Answer from the drawing. Dimensions are ordinates in mm from the lowest x, y and z of the part. A direction names the side the tool comes from. Give positions to 0.01 mm unless a question says otherwise; leave off trailing zeros. Order: outer loops, then holes, each group sorted by start corner. A loop starts at its lowest first (then second) coordinate and runs counter-clockwise, first axis right, second up. Notation, with made-up numbers: (67, 36.25) -> (76, 36.25) arc R31 ccw to (76, 69.25) -> close; hole circle Ø6 at (-20.75, 73). An arc over 180 degrees is marked (long way). Write item = value, one per line. Start each with the question number.
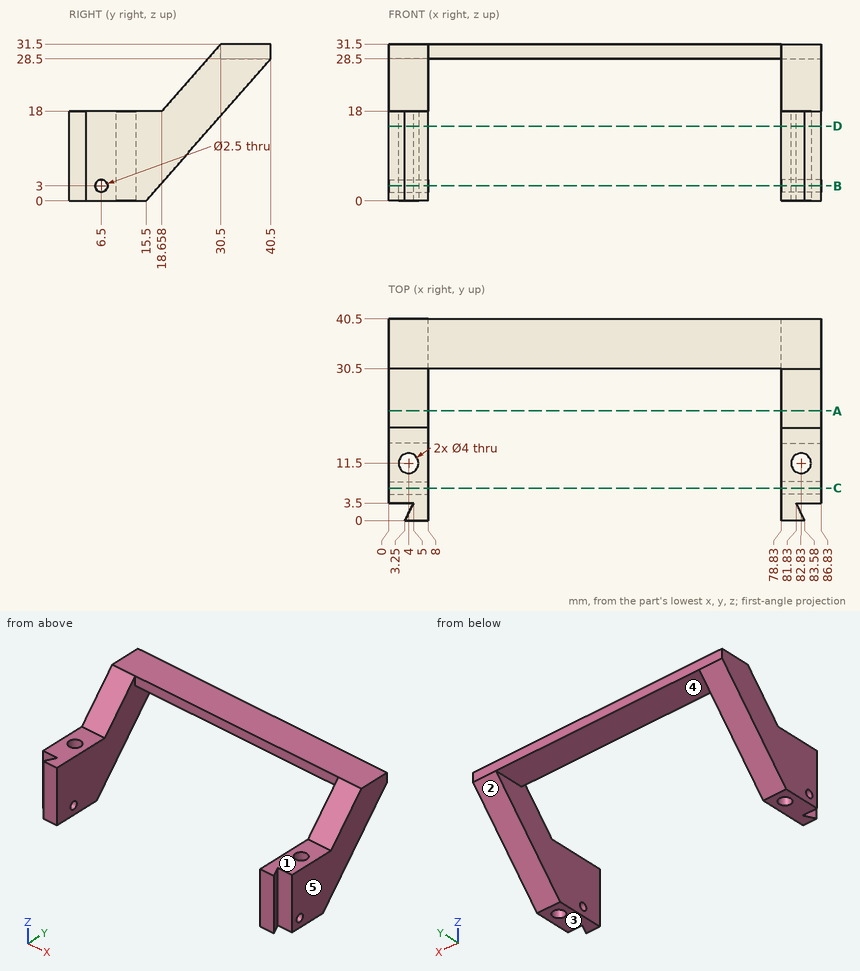
Item 1: Consider L1, parallel to Y at x = 82, z = 12; L2, parallel to X at y = 4, z = 2; L3, parallel to X at y = 12, z = 2. Determine where each line is inside the solid, lowest interval first. Write a range as from..to.
Item 2: A cutting plane is placed at A-A, the plane y = 22. Write down the section's boundary in (x, z), plus the area to 3 significant figures.
Item 3: A cutting plane is placed at C-C, the plane y = 6.5. Write down the section's boundary in (x, z).
Item 4: Flat-ended cylindrical pins translate along their axes: pin 1 (11 mm diameter, centred on x = 37.5, y = 34, fed in from -Z); pin 2 (6.5 mm diameter, centred on x = 84, y = 5.5, fed in from +Z); pin 3 (3.5 mm diameter, centred on x = 43.5, z = 29.5, fed in from -Y). Find the tip coordinate at first contact, or state that the pin passes through.
Item 5: Which of the six approach directions +Z, -Z, +X, -X, +Y, -Y give full straight-line access (tool end or side, diameter ignored) to the marked faces 1 and 2?
Item 6: A cutting plane is placed at B-B, the plane z = 3. Write down the section's boundary in (x, y), plus the area to 3 significant figures.
Item 7: The mould has two halves that part along X. Classify the marked faces 3, 4 and 5: +X half, -X half, draft (parallel to the pull), parting line (faces both ways), or undercut.
Item 8: A cutting plane is placed at D-D, the plane z = 15. Write down the section's boundary in (x, y).
Check values:
q1.L1 = 0..3.16, 3.5..9.68, 13.32..26.03
q1.L2 = 0..8, 78.83..86.83
q1.L3 = 0..2.06, 5.94..8, 78.83..80.89, 84.77..86.83
q2.outline = (0, 7.41) -> (8, 7.41) -> (8, 21.81) -> (0, 21.81) -> close; (78.83, 7.41) -> (86.83, 7.41) -> (86.83, 21.81) -> (78.83, 21.81) -> close
q2.area = 230 mm^2
q3.outline = (0, 0) -> (8, 0) -> (8, 1.75) -> (0, 1.75) -> close; (0, 4.25) -> (8, 4.25) -> (8, 18) -> (0, 18) -> close; (78.83, 0) -> (86.83, 0) -> (86.83, 1.75) -> (78.83, 1.75) -> close; (78.83, 4.25) -> (86.83, 4.25) -> (86.83, 18) -> (78.83, 18) -> close
q4.pin_1 = 28.5
q4.pin_2 = 18
q4.pin_3 = 30.5
q5.face_1 = +Z, +X, -X, -Y
q5.face_2 = -Z, +X, -X, +Y
q6.outline = (0, 3.5) -> (5, 3.5) -> (3.25, 0) -> (8, 0) -> (8, 5.25) -> (0, 5.25) -> close; (0, 7.75) -> (8, 7.75) -> (8, 18.13) -> (0, 18.13) -> close; (78.83, 0) -> (83.58, 0) -> (81.83, 3.5) -> (86.83, 3.5) -> (86.83, 5.25) -> (78.83, 5.25) -> close; (78.83, 7.75) -> (86.83, 7.75) -> (86.83, 18.13) -> (78.83, 18.13) -> close; hole circle Ø4 at (4, 11.5); hole circle Ø4 at (82.83, 11.5)
q6.area = 196 mm^2
q7.face_3 = draft
q7.face_4 = undercut
q7.face_5 = +X half
q8.outline = (0, 3.5) -> (5, 3.5) -> (3.25, 0) -> (8, 0) -> (8, 28.66) -> (0, 28.66) -> close; (78.83, 0) -> (83.58, 0) -> (81.83, 3.5) -> (86.83, 3.5) -> (86.83, 28.66) -> (78.83, 28.66) -> close; hole circle Ø4 at (4, 11.5); hole circle Ø4 at (82.83, 11.5)
